```python
from build123d import *

# Parameters (mm, degrees)
SKETCH1_W            = 40.7
SKETCH1_H            = 20.5
BOSS_EXTRUDE1_DEPTH  = 39.5
SKETCH2_R            = 3
BOSS_EXTRUDE2_DEPTH  = 4
SKETCH3_W            = 54.5
SKETCH3_H            = 20.5
BOSS_EXTRUDE3_DEPTH  = 3
CUT_EXTRUDE1_DEPTH   = 60.634386054
MIRROR2_COPY_1_DEPTH = 60.634386054


with BuildPart() as part:
    # Sketch1 → Boss-Extrude1 (new body)
    with BuildSketch(Plane(origin=(0, 0, 0), x_dir=(1, 0, 0), z_dir=(0, 1, 0))):
        with Locations((20.35, 10.25)):
            Rectangle(SKETCH1_W, SKETCH1_H)
    extrude(amount=BOSS_EXTRUDE1_DEPTH)

    # Sketch2 → Boss-Extrude2 (add)
    with BuildSketch(Plane(origin=(0, 39.5, 0), x_dir=(1, 0, 0), z_dir=(0, 1, 0))):
        with Locations(Location((10.25, 10.25, 0), (0, 0, 90))):
            Circle(SKETCH2_R)
    extrude(amount=BOSS_EXTRUDE2_DEPTH)

    # Sketch3 → Boss-Extrude3 (add)
    with BuildSketch(Plane(origin=(0, 29.5, 0), x_dir=(1, 0, 0), z_dir=(0, 1, 0))):
        with Locations((20.35, 10.25)):
            Rectangle(SKETCH3_W, SKETCH3_H)
    extrude(amount=BOSS_EXTRUDE3_DEPTH)

    # Sketch4 → Cut-Extrude1 (cut, through all)
    with BuildSketch(Plane(origin=(0, 29.5, 0), x_dir=(1, 0, 0), z_dir=(0, 1, 0))):
        with BuildLine():
            Line((-5.65, 17.25), (-6.9, 17.25))
            Line((-6.9, 17.25), (-6.9, 13.25))
            Line((-6.9, 13.25), (-5.65, 13.25))
            ThreePointArc((-5.65, 13.25), (-1.65, 15.25), (-5.65, 17.25))
        make_face()
    cut_extrude1 = extrude(amount=CUT_EXTRUDE1_DEPTH, mode=Mode.SUBTRACT)

    # Mirror1: Cut-Extrude1 across plane
    add(cut_extrude1.mirror(Plane(origin=(0, 0, -10.25), x_dir=(1, 0, 0), z_dir=(0, 0, -1))), mode=Mode.SUBTRACT)

    # Mirror2: Cut-Extrude1 across plane
    add(cut_extrude1.mirror(Plane(origin=(20.35, 0, 0), x_dir=(0, 0, 1), z_dir=(1, 0, 0))), mode=Mode.SUBTRACT)

    # Mirror2 copy 1 sketch → Mirror2 copy 1 (cut, through all)
    with BuildSketch(Plane(origin=(40.7, 29.5, -20.5), x_dir=(-1, 0, 0), z_dir=(0, 1, 0))):
        with BuildLine():
            Line((-5.65, 17.25), (-6.9, 17.25))
            Line((-6.9, 17.25), (-6.9, 13.25))
            Line((-6.9, 13.25), (-5.65, 13.25))
            ThreePointArc((-5.65, 13.25), (-1.65, 15.25), (-5.65, 17.25))
        make_face()
    extrude(amount=MIRROR2_COPY_1_DEPTH, mode=Mode.SUBTRACT)


solid = part.part
```
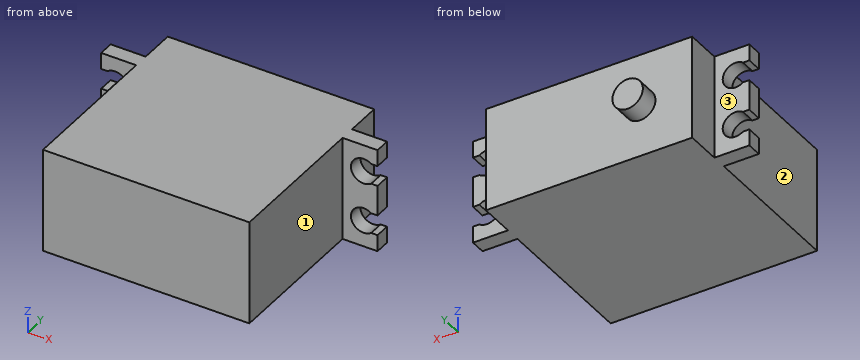
The listing builds one solid part. Answer for the finished solid, in the listing's coordinates (mm). Face numbers are marked on the shaded views. A direction names the side the tool comes from. Give positions to 0.01 mm unless a question says otherwise; leave off trailing zeros. Order: outer loops, then holes, each group sorted by start corner. A loop starts at its lowest first (then second) coordinate and runs counter-clockwise, first axis right, second up. Notation, with made-up numbers: (46, -29) - (78, -29) arc R23 cw to (78, 10) - close; hole circle Ø7 at (12, -24.75). An arc over 180 degrees is marked (long way). Use one line per item in the form item = value. Start each with the question number.
(1) Consider line 1 (Z direction, x = -4, y = 31); line 2 (X direction, y = 38, z = -19); line 3 (X direction, y = 30.2, z = -5.25). Determine where each line is inside the solid, lowest interval first. Write a range as from..to.
(2) Flat-ended cylindrical pins translate along their axes: pin 1 Ø8 at (x, z) = (44.85, -15.25) entering from -Y; pin 2 Ø12 at (y, z) = (7.5, -7) entering from +X; pin 3 Ø5 at (x, z) = (37, -11.5) entering from +Y; pin 4 Ø4 at (x, z) = (-4.15, -5.25) entering from +Y. Find the tip coordinate at first contact, or state that the pin passes through.
(3) A cutting plane is placed at A-A, the plane x = -4.15. Write down the section's boundary in (y, z).
(4) A cutting plane is placed at B-B, the plane z = -10.25. Write down the section's boundary in (x, y), then the cut area to 3 significant figures.
(5) A cutting plane is placed at C-C, the plane y = 24. Write down the section's boundary in (x, z).
(6) A cutting plane is placed at D-D, the plane x = 11.5. Write down the section's boundary in (y, z).
(7) For the marked faces 1, 2 and 3, determine the directions among +Z, -Z, +X, -X, +Y, -Y from which every point of the face is accessible in a straight line to the end or side of a thin tool.
Ans:
q1.line_1 = -20.5..-17.75, -12.75..-7.75, -2.75..0
q1.line_2 = 0..40.7
q1.line_3 = -1.65..42.35
q2.pin_1 = 29.5
q2.pin_2 = 40.7
q2.pin_3 = 39.5
q2.pin_4 = through
q3.outline = (29.5, -20.5) - (32.5, -20.5) - (32.5, -17.75) - (29.5, -17.75) - close; (29.5, -12.75) - (32.5, -12.75) - (32.5, -7.75) - (29.5, -7.75) - close; (29.5, -2.75) - (32.5, -2.75) - (32.5, 0) - (29.5, 0) - close
q4.outline = (-6.9, 29.5) - (0, 29.5) - (0, 0) - (40.7, 0) - (40.7, 29.5) - (47.6, 29.5) - (47.6, 32.5) - (40.7, 32.5) - (40.7, 39.5) - (13.25, 39.5) - (13.25, 43.5) - (7.25, 43.5) - (7.25, 39.5) - (0, 39.5) - (0, 32.5) - (-6.9, 32.5) - close
q4.area = 1,670 mm^2
q5.outline = (0, -20.5) - (40.7, -20.5) - (40.7, 0) - (0, 0) - close
q6.outline = (0, -20.5) - (39.5, -20.5) - (39.5, -12.98) - (43.5, -12.98) - (43.5, -7.52) - (39.5, -7.52) - (39.5, 0) - (0, 0) - close
q7.face_1 = +Z, -Z, +X, -Y
q7.face_2 = +Z, -Z, -X, -Y
q7.face_3 = +Z, -Z, -X, +Y
